The drawing under review shows one solid part. Ordinate dimensions are in mm from its lowest x, y, z. Round coordinates to 2 decimals unless told otherwise and drop trailing zeros. Order: outer loops, then holes, each group sorted by start corner. A loop starts at its lowest first (then second) coordinate and runs counter-clockwise, first axis right, second up.
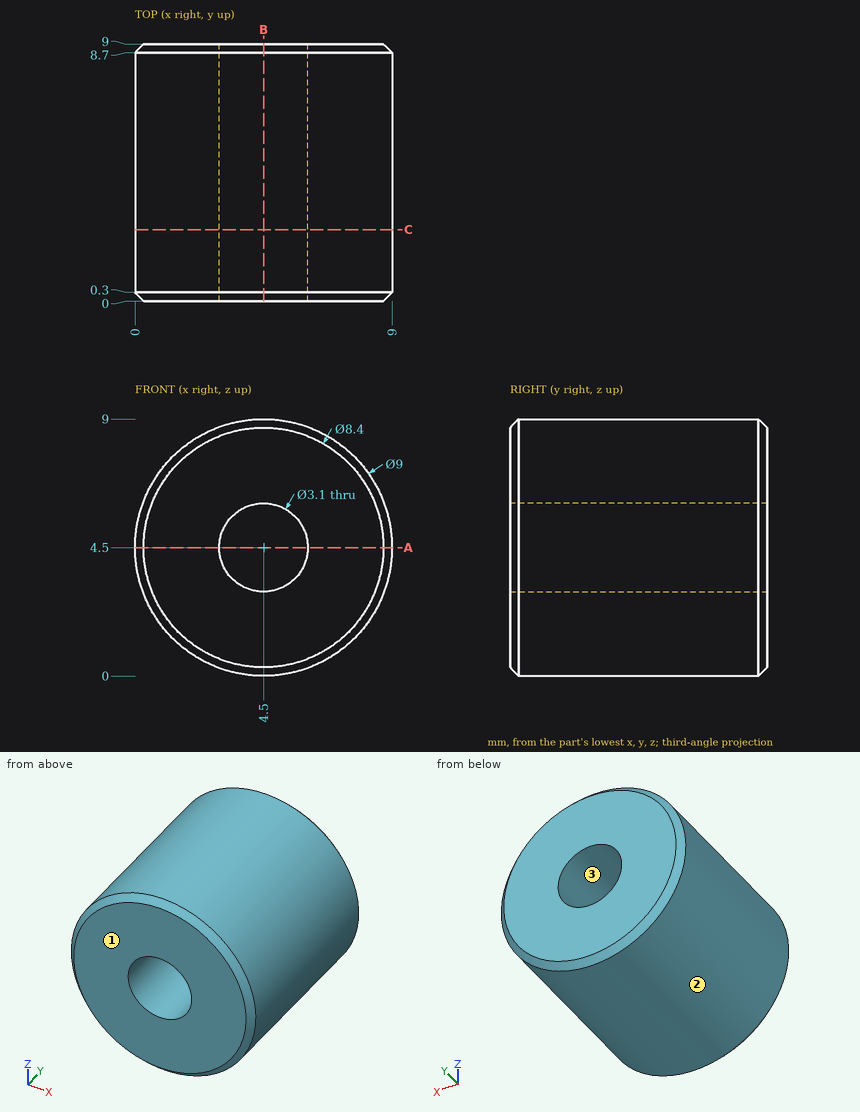
Q1. Take a section at A-A, the plane z = 4.5. State the section outline as (x, y) points, plus the area to 3 significant figures.
Q2. Mouldability with a two-part tool opening along Z and no side actions: class the marked faces 1, 2 and 3 as +Z half, -Z half, draft (parallel to the pull), parting line (faces both ways), or undercut.
Q3. Take a section at B-B, the plane x = 4.5. State the section outline as (y, z) points.
Q4. Wall thickness on line 1 (X direction, y = 5, z = 4.5); line 2 (Z direction, x = 3.25, y = 2): over which ranges is each line inside the solid? List them lowest first.
Q5. Take a section at C-C, the plane y = 2.5. State the section outline as (x, z) points, plus the area to 3 significant figures.
Q6. Clearance check with flat-ended pins moving along their axes: pin 1 (1.9 mm diameter, centred on x = 4.5, z = 4.5, fed in from +Y); pin 2 (2 mm diameter, centred on x = 8, y = 7, fed in from +Z). State where each tip first meets the part, or that it passes through.
Working result:
1. outline: (0, 0.3) - (0.3, 0) - (2.95, 0) - (2.95, 9) - (0.3, 9) - (0, 8.7) - close; (6.05, 0) - (8.7, 0) - (9, 0.3) - (9, 8.7) - (8.7, 9) - (6.05, 9) - close
1. area: 52.9 mm2
2. face 1: draft
2. face 2: parting line
2. face 3: undercut
3. outline: (0, 0.3) - (0.3, 0) - (8.7, 0) - (9, 0.3) - (9, 2.95) - (0, 2.95) - close; (0, 6.05) - (9, 6.05) - (9, 8.7) - (8.7, 9) - (0.3, 9) - (0, 8.7) - close
4. line 1: x = 0 to 2.95, 6.05 to 9
4. line 2: z = 0.18 to 3.58, 5.42 to 8.82
5. outline: circle Ø9 at (4.5, 4.5); hole circle Ø3.1 at (4.5, 4.5)
5. area: 56.1 mm2
6. pin 1: passes through
6. pin 2: stops at z = 8.24
